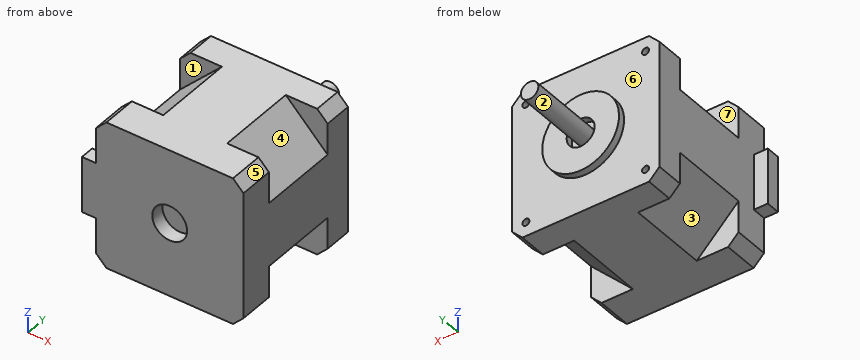
from build123d import *

# Parameters (mm, degrees)
BOSS_EXTRUDE1_START       = -22
BOSS_EXTRUDE1_DEPTH       = 8
BOSS_EXTRUDE3_DEPTH       = 23
BOSS_EXTRUDE4_DEPTH       = 6
SKETCH4_R                 = 11
SKETCH4_R_2               = 4
BOSS_EXTRUDE5_DEPTH       = 2
SKETCH5_R                 = 2.5
BOSS_EXTRUDE6_DEPTH       = 22
F_2_0MM_DOWEL_HOLE1_D     = 2
F_2_0MM_DOWEL_HOLE1_DEPTH = 5
F_2_0MM_DOWEL_HOLE1_TIP   = 0.600860619
SKETCH8_R                 = 5
SKETCH8_W                 = 4
SKETCH8_H                 = 16
BOSS_EXTRUDE7_DEPTH       = 4


with BuildPart() as part:
    # Sketch1 → Boss-Extrude1 (new body)
    with BuildSketch(Plane(origin=(0, 0, 0), x_dir=(1, 0, 0), z_dir=(0, 1, 0)).offset(BOSS_EXTRUDE1_START)):
        Polygon((-18.15, 21.15), (-21.15, 18.15), (-21.15, -18.15), (-18.15, -21.15), (18.15, -21.15), (21.15, -18.15), (21.15, 18.15), (18.15, 21.15), align=None)
    extrude(amount=-BOSS_EXTRUDE1_DEPTH)

    # Sketch2 → Boss-Extrude3 (add)
    with BuildSketch(Plane(origin=(0, -30, 0), x_dir=(-1, 0, 0), z_dir=(0, -1, 0))):
        Polygon((-21.15, 9.15), (-9.15, 21.15), (9.15, 21.15), (21.15, 9.15), (21.15, -9.15), (9.15, -21.15), (-9.15, -21.15), (-21.15, -9.15), align=None)
    extrude(amount=BOSS_EXTRUDE3_DEPTH)

    # Sketch3 → Boss-Extrude4 (add)
    with BuildSketch(Plane(origin=(0, -53, 0), x_dir=(-1, 0, 0), z_dir=(0, -1, 0))):
        Polygon((-18.15, 21.15), (-21.15, 18.15), (-21.15, -18.15), (-18.15, -21.15), (18.15, -21.15), (21.15, -18.15), (21.15, 18.15), (18.15, 21.15), align=None)
    extrude(amount=BOSS_EXTRUDE4_DEPTH)

    # Sketch4 → Boss-Extrude5 (add)
    with BuildSketch(Plane(origin=(0, -22, 0), x_dir=(-1, 0, 0), z_dir=(0, 1, 0))):
        with Locations(Location((0, 0, 0), (0, 0, 90))):
            Circle(SKETCH4_R)
        with Locations(Location((0, 0, 0), (0, 0, 90))):
            Circle(SKETCH4_R_2, mode=Mode.SUBTRACT)
    extrude(amount=BOSS_EXTRUDE5_DEPTH)

    # Sketch5 → Boss-Extrude6 (add)
    with BuildSketch(Plane(origin=(0, -22, 0), x_dir=(-1, 0, 0), z_dir=(0, 1, 0))):
        with Locations(Location((0, 0, 0), (0, 0, 90))):
            Circle(SKETCH5_R)
    extrude(amount=BOSS_EXTRUDE6_DEPTH)

    # Ø2.0mm Dowel Hole1
    with Locations(Plane(origin=(0, -22, 0), x_dir=(1, 0, 0), z_dir=(0, 1, 0))):
        with Locations((-17.15, 17.15), (-17.15, -17.15), (17.15, -17.15), (17.15, 17.15)):
            Hole(F_2_0MM_DOWEL_HOLE1_D / 2, depth=F_2_0MM_DOWEL_HOLE1_DEPTH)
            with Locations((0, 0, -(F_2_0MM_DOWEL_HOLE1_DEPTH + F_2_0MM_DOWEL_HOLE1_TIP / 2))):  # 118° drill point
                Cone(0, F_2_0MM_DOWEL_HOLE1_D / 2, F_2_0MM_DOWEL_HOLE1_TIP, mode=Mode.SUBTRACT)

    # Sketch8 → Boss-Extrude7 (add)
    # profile 1 of 2: a face of its own
    with BuildSketch(Plane.XZ.offset(59)):
        Polygon((-21.15, -18.15), (-18.15, -21.15), (18.15, -21.15), (21.15, -18.15), (21.15, 18.15), (18.15, 21.15), (-18.15, 21.15), (-21.15, 18.15), align=None)
        with Locations(Location((0, 0, 0), (0, 0, 270))):
            Circle(SKETCH8_R, mode=Mode.SUBTRACT)
    # profile 2 of 2: a face of its own
    with BuildSketch(Plane.XZ.offset(59)):
        with Locations((-23.15, 0)):
            Rectangle(SKETCH8_W, SKETCH8_H)
    extrude(amount=BOSS_EXTRUDE7_DEPTH)


solid = part.part
Check sheet for the modelled part. Datum: model origin and axes. Units: mm. Face numbers are marked on the shaded views. A direction names the side the tool comes from. Coordinates: 2 decimals unless noted, no trailing zeros. Loops run counter-clockwise (first coordinate to the right, second up) from the corner with the lowest first, then second, coordinate; pieces in that order, holes last. Notation, with made-up numbers: (-22, 5) -> (23, 5) arc R28 ccw to (23, 29) -> close; hole circle Ø2 at (84.5, 66). An arc over 180 degrees is marked (long way). Write item = value, one per line. Start each with the question number.
1. Tool access check on the marked faces 1, 2, 3 and 4. Record the directions out of +Z, -Z, +X, -X, +Y, -Y that give a thin tool (end or side, any length) a straight path to the whole face; none if there is none.
2. Draft check along Y on the marked faces 5, 6 and 7. Enter one of: released by +Y, released by -Y, zero draft, split by the parting line, or undercut.
3. Section check B-B on x = 0. Record the cut outline in (y, z).
4. Section check D-D on y = -40. Record the cut outline in (x, z).
5. Section check A-A on y = -25.5. Record the cut outline in (x, z).
6. Section check C-C on z = 14. Record the cut outline in (x, y).
7. Material ranges on line 1 (X direction, y = -20.45, z = 0); line 2 (X direction, y = -23, z = 17), recorded low to high.
8. Depth check by flat-ended pin: P1, Ø4, axis at x = -14.5, z = 6, coming from the +Y side; P2, Ø2, axis at x = -23.5, z = 3, coming from the +Y side; P3, Ø11, axis at y = -40, z = -1, coming from the -X side. Enter the tip coordinate at first touch or a pass-through.
Responses:
q1.face_1 = +Z, -X
q1.face_2 = +Y
q1.face_3 = -Z, -X
q1.face_4 = +Z, +X
q2.face_5 = zero draft
q2.face_6 = released by +Y
q2.face_7 = undercut
q3.outline = (-63, -21.15) -> (-22, -21.15) -> (-22, -11) -> (-20, -11) -> (-20, -4) -> (-22, -4) -> (-22, -2.5) -> (0, -2.5) -> (0, 2.5) -> (-22, 2.5) -> (-22, 4) -> (-20, 4) -> (-20, 11) -> (-22, 11) -> (-22, 21.15) -> (-63, 21.15) -> (-63, 5) -> (-59, 5) -> (-59, -5) -> (-63, -5) -> close
q4.outline = (-21.15, -9.15) -> (-9.15, -21.15) -> (9.15, -21.15) -> (21.15, -9.15) -> (21.15, 9.15) -> (9.15, 21.15) -> (-9.15, 21.15) -> (-21.15, 9.15) -> close
q5.outline = (-21.15, -18.15) -> (-18.15, -21.15) -> (18.15, -21.15) -> (21.15, -18.15) -> (21.15, 18.15) -> (18.15, 21.15) -> (-18.15, 21.15) -> (-21.15, 18.15) -> close; hole circle Ø2 at (-17.15, -17.15); hole circle Ø2 at (-17.15, 17.15); hole circle Ø2 at (17.15, -17.15); hole circle Ø2 at (17.15, 17.15)
q6.outline = (-21.15, -63) -> (21.15, -63) -> (21.15, -53) -> (16.3, -53) -> (16.3, -30) -> (21.15, -30) -> (21.15, -22) -> (-21.15, -22) -> (-21.15, -30) -> (-16.3, -30) -> (-16.3, -53) -> (-21.15, -53) -> close
q7.line_1 = -11 to -4, -2.5 to 2.5, 4 to 11
q7.line_2 = -21.15 to -18.14, -16.16 to 16.16, 18.14 to 21.15
q8.P1 = -22
q8.P2 = -59
q8.P3 = -21.15
